The listing builds one solid part. Answer for the finished solid, in the listing's coordinates (mm). Face numbers are marked on the shaded views. A direction names the side the tool comes from. Coordinates: 2 decimals unless noted, no trailing zeros. Order: outer loops, then holes, each group sorted by start corner. A loop starts at its lowest first (then second) coordinate and runs counter-clockwise, first axis right, second up. Notation, with made-up numbers: (-4, -26.75) -> (14, -26.75) arc R18 ccw to (14, 5.25) -> close; hole circle Ø11 at (-37, 36). An arc over 180 degrees is marked (long way). Return JSON: item names as keys, results as strings.
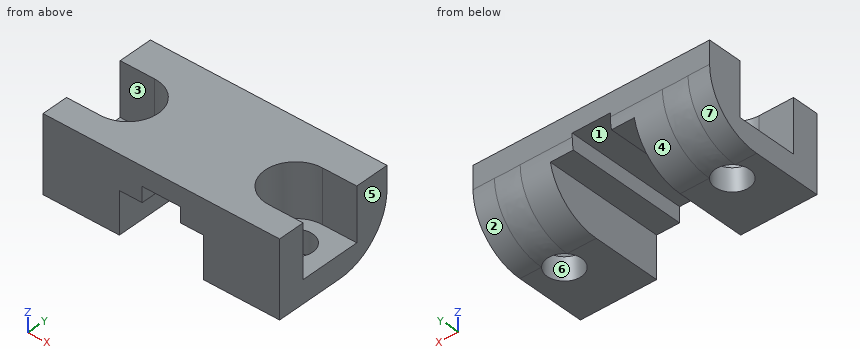
Solid Edge part; units mm, degrees
sketch "Sketch1" plane through (0, 0, 1.5849) normal (0, 0, 1) x (1, 0, 0)
  line L0 (15.5, 101) -> (-15.5, 101)
  line L1 (-15.5, 101) -> (-15.5, 117)
  line L2 (-15.5, 117) -> (15.5, 117)
  line L3 (15.5, 101) -> (15.5, 117)
extrude "Protrusion1" add sketch "Sketch1" along normal blind 10
sketch "Sketch2" plane through (0, 0, 1.5849) normal (0, 0, 1) x (1, 0, 0)
  circle A0 centre (11, 108.5) radius 2.25
  circle A1 centre (-11, 108.5) radius 2.25
extrude "Cutout1" cut sketch "Sketch2" along normal up to next
sketch "Sketch3" plane through (0, 101, 13.75) normal (0, -1, 0) x (1, 0, 0)
  line L0 (2.5, -6.6651) -> (5.5112, -6.6651)
  line L1 (5.5112, -12.1651) -> (5.5112, -6.6651)
  line L2 (-5.4918, -12.1651) -> (5.5112, -12.1651)
  line L3 (-5.4918, -6.6651) -> (-5.4918, -12.1651)
  line L4 (-5.4918, -6.6651) -> (-2.5, -6.6651)
  line L5 (-2.5, -4.6651) -> (-2.5, -6.6651)
  line L6 (2.5, -4.6651) -> (-2.5, -4.6651)
  line L7 (2.5, -4.6651) -> (2.5, -6.6651)
extrude "Cutout2" cut sketch "Sketch3" against normal up to next
sketch "Sketch4" plane through (0, 109, 11.5849) normal (0, 0, 1) x (1, 0, 0)
  line L0 (-15.5, 3.5) -> (-15.5, -4.5)
  line L1 (-11, -4.5) -> (-15.5, -4.5)
  line L2 (-11, 3.5) -> (-15.5, 3.5)
  arc A0 (-11, 3.5) -> (-11, -4.5) centre (-11, -0.5) cw
  line L3 (11, 3.5) -> (15.5, 3.5)
  line L4 (15.5, 3.5) -> (15.5, -4.5)
  line L5 (11, -4.5) -> (15.5, -4.5)
  arc A1 (11, -4.5) -> (11, 3.5) centre (11, -0.5) cw
extrude "ExtrudedCutout_3" cut sketch "Sketch4" against normal blind 7
fillet "Round_1" radius 7 2 edges at (10.5056, 117, 1.5849) (-10.4959, 117, 1.5849)
1. Each of these flat-tipped pins is pushed along its axis until it touches: pin 1 Ø1 at (y, z) = (110, 8.5) entering from +X; pin 2 Ø0.6 at (y, z) = (105.5, 8.5) entering from -X; pin 3 Ø4 at (x, y) = (-1, 109.5) entering from -Z. Where does it stop, or does it pass through?
Answer block:
{"pin 1": "stops at x = 7.54", "pin 2": "stops at x = -8.74", "pin 3": "stops at z = 7.08"}
2. For the marked faces 1, 2, 3 and 4, determine the directions among +Z, -Z, +X, -X, +Y, -Y from which every point of the face is accessible in a straight line to the end or side of a thin tool.
Answer block:
{"face 1": "-Z, +Y, -Y", "face 2": "-Z, +X, +Y", "face 3": "+Z, -X", "face 4": "-Z, +Y"}
3. Consider line 1 (X direction, y = 108.5, z = 2.9); line 2 (X direction, y = 102.75, z = 8.5); line 3 (X direction, y = 103.5, z = 3.25). Determine where each line is inside the solid, lowest interval first. Write a range as from..to.
Answer block:
{"line 1": "x = -15.5..-13.25, -8.75..-5.49, 5.51..8.75, 13.25..15.5", "line 2": "x = -15.5..-2.5, 2.5..15.5", "line 3": "x = -15.5..-5.49, 5.51..15.5"}
4. The part is cut by section C-C on z = 9.75. Give the vertices of the cut face in (x, y).
Answer block:
{"outline": "(-15.5, 101) -> (15.5, 101) -> (15.5, 104.5) -> (11, 104.5) arc R4 cw to (11, 112.5) -> (15.5, 112.5) -> (15.5, 117) -> (-15.5, 117) -> (-15.5, 112.5) -> (-11, 112.5) arc R4 cw to (-11, 104.5) -> (-15.5, 104.5) -> close"}
5. The part is cut by section D-D on z = 3.5. Give the number of separate pieces and of enclosed holes in the cut face, and give its area (3 significant figures).
Answer block:
{"separate pieces": "2", "enclosed holes": "2", "area": "245 mm2"}
6. Determine the mould class of the marked faces 5, 6 and 7 for opening direction X: pulls with the +X half, pulls with the -X half, needs draft (parallel to the pull), parting line crosses it, or undercut.
Answer block:
{"face 5": "pulls with the +X half", "face 6": "undercut", "face 7": "needs draft"}
7. The part is cut by section B-B on x = 5. Give the vertices of the cut face in (y, z), and give its area (3 significant figures).
Answer block:
{"outline": "(101, 7.08) -> (116.84, 7.08) arc R7 ccw to (117, 8.58) -> (117, 11.58) -> (101, 11.58) -> close", "area": "71.9 mm2"}
8. The part is cut by section A-A on y = 108.5. Give the vertices of the cut face in (x, z).
Answer block:
{"outline": "(-15.5, 1.58) -> (-13.25, 1.58) -> (-13.25, 4.58) -> (-15.5, 4.58) -> close; (-8.75, 1.58) -> (-5.49, 1.58) -> (-5.49, 7.08) -> (-2.5, 7.08) -> (-2.5, 9.08) -> (2.5, 9.08) -> (2.5, 7.08) -> (5.51, 7.08) -> (5.51, 1.58) -> (8.75, 1.58) -> (8.75, 4.58) -> (7, 4.58) -> (7, 11.58) -> (-7, 11.58) -> (-7, 4.58) -> (-8.75, 4.58) -> close; (13.25, 1.58) -> (15.5, 1.58) -> (15.5, 4.58) -> (13.25, 4.58) -> close"}
